Part model, mm, in its own coordinate system. A direction names the side the tool comes from. Give positions to 0.01 mm unless a question says otherwise; leave off trailing zeros. Order: outer loops, then holes, each group sorted by start corner. A loop starts at its lowest first (then second) coordinate and runs counter-clockwise, first axis right, second up. Notation, with made-up numbers: (25, 13.25) - (49, 13.25) arc R16 ccw to (49, 33.25) - close; hole circle Ø11 at (-31, 57.5). An arc over 180 degrees is marked (long way). One line per item, written item: value.
Autodesk Inventor part; units mm, degrees
ref_plane "YZ Plane" through (0, 0, 0) normal (1, 0, 0) x (0, 1, 0)
ref_plane "XZ Plane" through (0, 0, 0) normal (0, 1, 0) x (-1, 0, 0)
ref_plane "XY Plane" through (0, 0, 0) normal (0, 0, 1) x (1, 0, 0)
sketch "Esquisse1" plane through (0, 0, 0) normal (0, 1, 0) x (-1, 0, 0)
  line L0 (35, 35) -> (35, 14)
  line L1 (35, 14) -> (42, 10)
  line L2 (42, 10) -> (42, 0)
  line L3 (35, 35) -> (0, 0)
  line L4 (42, 0) -> (0, 0) construction
  line L5 (35, -35) -> (35, -14)
  line L6 (35, -14) -> (42, -10)
  line L7 (42, -10) -> (42, 0)
  line L8 (35, -35) -> (0, 0)
  line L9 (38.5, -12) -> (38.5, 12) construction
  circle A0 centre (38.5, 0) radius 2.15
  circle A1 centre (38.5, 6) radius 2.15
  circle A2 centre (38.5, -6) radius 2.15
  dimension "d0" = 90
  dimension "d1" = 70
  dimension "d4" = 6
  dimension "d11" = 6
  dimension "d16" = 4.3
  dimension "d17" = 20
  dimension "d18" = 4
  dimension "d19" = 7
extrude "Extrusion1" add sketch "Esquisse1" along normal blind 3
pattern_circular "Réseau circulaire1" count 4 over 360 about axis through (0, 0, 0) along (0, 1, 0) of "Extrusion1"
ref_plane "Plan de construction2" through (0, 0, -14) normal (1, 0, 0) x (0, 0, -1)
ref_plane "Plan de construction3" through (-14, 0, 0) normal (0, 0, -1) x (-1, 0, 0)
chamfer "Chanfrein1" distance 10 angle 45 4 edges at (-35, 1.5, -35) (-35, 1.5, 35) (35, 1.5, -35) (35, 1.5, 35)
sketch "Esquisse3" plane through (0, 0, 0) normal (0, -1, 0) x (1, 0, 0)
  circle A0 centre (0, 38.5) radius 2.15 construction
  circle A1 centre (6, 38.5) radius 2.15 construction
  circle A2 centre (-6, 38.5) radius 2.15 construction
  circle A3 centre (38.5, 6) radius 2.15 construction
  circle A4 centre (38.5, -6) radius 2.15 construction
  circle A5 centre (38.5, 0) radius 2.15 construction
  circle A6 centre (6, -38.5) radius 2.15 construction
  circle A7 centre (-6, -38.5) radius 2.15 construction
  circle A8 centre (0, -38.5) radius 2.15 construction
  circle A9 centre (-38.5, -6) radius 2.15 construction
  circle A10 centre (-38.5, 6) radius 2.15 construction
  circle A11 centre (-38.5, 0) radius 2.15 construction
  line L0 (-35, 25) -> (-35, 14) construction
  line L1 (-35, 14) -> (-42, 10) construction
  line L2 (-42, 10) -> (-42, -10) construction
  line L3 (-42, -10) -> (-35, -14) construction
  line L4 (-35, -14) -> (-35, -25) construction
  line L5 (-25, -35) -> (-14, -35) construction
  line L6 (-14, -35) -> (-10, -42) construction
  line L7 (-10, -42) -> (10, -42) construction
  line L8 (10, -42) -> (14, -35) construction
  line L9 (14, -35) -> (25, -35) construction
  line L10 (35, -25) -> (35, -14) construction
  line L11 (35, -14) -> (42, -10) construction
  line L12 (42, -10) -> (42, 10) construction
  line L13 (42, 10) -> (35, 14) construction
  line L14 (35, 14) -> (35, 25) construction
  line L15 (25, 35) -> (14, 35) construction
  line L16 (14, 35) -> (10, 42) construction
  line L17 (10, 42) -> (-10, 42) construction
  line L18 (-10, 42) -> (-14, 35) construction
  line L19 (-14, 35) -> (-25, 35) construction
  line L20 (-51.72, -12.8291) -> (-12.8291, -51.72)
  line L21 (-12.8291, -51.72) -> (-10, -42)
  line L22 (-42, -10) -> (-51.72, -12.8291)
  line L23 (-35, -14) -> (-42, -10)
  line L24 (-42, -10) -> (-35, -14)
  line L25 (-10, -42) -> (-14, -35)
  line L26 (-14, -35) -> (-10, -42)
  line L27 (25, 35) -> (35, 25)
  line L28 (-35, 25) -> (-25, 35)
  line L29 (-25, -35) -> (-35, -25)
  line L30 (35, -25) -> (25, -35)
  line L31 (-14, -35) -> (-35, -14)
  point P0 (0, 0)
  dimension "d32" = 135
  dimension "d33" = 55
extrude "Extrusion3" add sketch "Esquisse3" against normal blind 3
sketch "Esquisse4" plane through (-51.72, 0, -12.8291) normal (-0.7071068, 0, -0.7071068) x (-0.7071068, 0, 0.7071068)
  line L0 (0, 0) -> (-55, 0) construction
  line L1 (0, 0) -> (0, 3) construction
  line L2 (-55, 3) -> (0, 3) construction
  line L3 (-55, 0) -> (-55, 3) construction
  line L4 (0, 0) -> (-55, 0)
  line L5 (-55, 0) -> (-55, 24)
  line L6 (-55, 24) -> (0, 24)
  line L7 (0, 24) -> (0, 0)
  point P0 (-27.5, 0)
  dimension "d36" = 24
extrude "Extrusion4" add sketch "Esquisse4" along normal blind 3
sketch "Esquisse5" plane through (-53.8413, 0, -14.9504) normal (-0.7071068, 0, -0.7071068) x (-0.7071068, 0, 0.7071068)
  line L0 (-55, 0) -> (0, 0) construction
  line L1 (0, 0) -> (0, 24) construction
  line L2 (0, 24) -> (-55, 24) construction
  line L3 (-55, 24) -> (-55, 0) construction
  line L4 (0, 0) -> (0, 24) construction
  line L5 (0, 9.2801) -> (-55, 9.2801) construction
  circle A0 centre (-15.1412, 9.2801) radius 7.3571
  line L6 (-27.5, 0) -> (-27.5, 24) construction
  circle A1 centre (-39.8588, 9.2801) radius 7.3571
extrude "Extrusion5" cut sketch "Esquisse5" against normal blind 1
pattern_circular "Réseau circulaire2" count 4 over 360 about axis through (0, 0, 0) along (0, -1, 0) of "Extrusion3", "Extrusion4"
fillet "Congé1" radius 3 2 edges at (-34.3959, 0, 34.3959) (34.3959, 0, -34.3959)
sketch "Esquisse6" plane through (0, 0, 0) normal (0, -1, 0) x (1, 0, 0)
  line L0 (51.72, -12.8291) -> (12.8291, -51.72) construction
  line L1 (51.72, -12.8291) -> (42, -10) construction
  line L2 (42, -10) -> (42, 10) construction
  line L3 (42, 10) -> (51.72, 12.8291) construction
  line L4 (51.72, 12.8291) -> (53.8413, 14.9504) construction
  line L5 (14.9504, 53.8413) -> (53.8413, 14.9504) construction
  line L6 (12.8291, 51.72) -> (14.9504, 53.8413) construction
  line L7 (12.8291, 51.72) -> (10, 42) construction
  line L8 (10, 42) -> (-10, 42) construction
  line L9 (-10, 42) -> (-12.8291, 51.72) construction
  line L10 (-51.72, 12.8291) -> (-12.8291, 51.72) construction
  line L11 (-51.72, 12.8291) -> (-42, 10) construction
  line L12 (-42, 10) -> (-42, -10) construction
  line L13 (-42, -10) -> (-51.72, -12.8291) construction
  line L14 (-51.72, -12.8291) -> (-53.8413, -14.9504) construction
  line L15 (-14.9504, -53.8413) -> (-53.8413, -14.9504) construction
  line L16 (-12.8291, -51.72) -> (-14.9504, -53.8413) construction
  line L17 (-12.8291, -51.72) -> (-10, -42) construction
  line L18 (-10, -42) -> (10, -42) construction
  line L19 (10, -42) -> (12.8291, -51.72) construction
  circle A0 centre (0, 38.5) radius 2.15 construction
  circle A1 centre (6, 38.5) radius 2.15 construction
  circle A2 centre (-6, 38.5) radius 2.15 construction
  circle A3 centre (38.5, 6) radius 2.15 construction
  circle A4 centre (38.5, -6) radius 2.15 construction
  circle A5 centre (38.5, 0) radius 2.15 construction
  circle A6 centre (6, -38.5) radius 2.15 construction
  circle A7 centre (-6, -38.5) radius 2.15 construction
  circle A8 centre (0, -38.5) radius 2.15 construction
  circle A9 centre (-38.5, -6) radius 2.15 construction
  circle A10 centre (-38.5, 6) radius 2.15 construction
  circle A11 centre (-38.5, 0) radius 2.15 construction
  line L20 (14.9504, -53.8413) -> (53.8413, -14.9504) construction
  line L21 (22.0215, -46.7702) -> (-16.8694, -7.8793)
  line L22 (-16.8694, -7.8793) -> (7.8793, 16.8694)
  line L23 (7.8793, 16.8694) -> (46.7702, -22.0215)
  line L24 (46.7702, -22.0215) -> (22.0215, -46.7702)
  line L25 (-16.8694, -7.8793) -> (-13.3339, -11.4149) construction
  line L26 (-13.3339, -11.4149) -> (11.4149, 13.3339) construction
  line L27 (11.4149, 13.3339) -> (7.8793, 16.8694) construction
  line L28 (-4.495, 4.495) -> (34.3959, -34.3959) construction
  line L29 (-13.3339, -11.4149) -> (-30.7818, -28.8628) construction
  circle A12 centre (-15.4552, -13.5362) radius 1.7
  circle A13 centre (-18.9907, -17.0717) radius 1.7
  circle A14 centre (13.5362, 15.4552) radius 1.7
  circle A15 centre (17.0717, 18.9907) radius 1.7
  point P0 (0, 0)
  dimension "d48" = 35
  dimension "d49" = 55
  dimension "d54" = 35
  dimension "d69" = 5
  dimension "d70" = 3
  dimension "d71" = 3.4
  dimension "d74" = 5
extrude "Extrusion6" cut sketch "Esquisse6" against normal through all contours L21 L22 L23 L24 keep common part
sketch "Esquisse7" plane through (19.9002, 3, -44.6489) normal (-0.7071068, 0, -0.7071068) x (-0.7071068, 0, 0.7071068)
  circle A0 centre (47, -5.5) radius 3.5
  line L0 (47, -3) -> (47, -5.5) construction
  line L1 (0, -3) -> (52, -3) construction
  point P0 (45.6431, -3)
  point P1 (47, -3)
  dimension "d97" = 2.5
  dimension "d98" = 7
extrude "Extrusion7" add sketch "Esquisse7" against normal blind 35
sketch "Esquisse8" plane through (19.9002, 3, -44.6489) normal (-0.7071068, 0, -0.7071068) x (-0.7071068, 0, 0.7071068)
  arc A0 (43.5, -3) -> (50.5, -3) centre (47, -3) ccw
  line L0 (49.4495, -3) -> (52, -3)
  line L1 (52, -3) -> (52, 0)
  line L2 (52, 0) -> (0, 0)
  line L3 (0, 0) -> (0, 21)
  line L4 (0, 21) -> (-3, 21)
  line L5 (-3, 21) -> (-3, 0)
  arc A1 (-3, 0) -> (0, -3) centre (0, 0) ccw
  line L6 (0, -3) -> (44.5505, -3)
  arc A2 (44.5505, -3) -> (49.4495, -3) centre (47, -5.5) ccw
  arc A3 (44.5505, -3) -> (49.4495, -3) centre (47, -5.5) ccw
  circle A4 centre (47, -5.5) radius 2.3
  point P0 (45.6431, -3)
  dimension "d99" = 4.6
extrude "Extrusion8" cut sketch "Esquisse8" against normal through all contours A4 A0 | A0 A4
sketch "Esquisse11" plane through (19.9002, 3, -44.6489) normal (-0.7071068, 0, -0.7071068) x (-0.7071068, 0, 0.7071068)
  line L0 (49.4495, -3) -> (52, -3)
  line L1 (52, -3) -> (52, 0)
  line L2 (52, 0) -> (0, 0)
  line L3 (0, 0) -> (0, 21)
  line L4 (0, 21) -> (-3, 21)
  line L5 (-3, 21) -> (-3, 0)
  arc A0 (-3, 0) -> (0, -3) centre (0, 0) ccw
  line L6 (0, -3) -> (44.5505, -3)
  arc A1 (44.5505, -3) -> (49.4495, -3) centre (47, -5.5) ccw
  line L7 (49.4495, -3) -> (49, 0) construction
  line L8 (52, 0) -> (0, 0)
  line L9 (49, 0) -> (42, 0) construction
  spline S0 degree 2 poles (49.4495, -3) (49, 0) (42, 0) knots 1 1 1 2 2 2
  point P0 (45.6431, -3)
  dimension "d100" = 3
  dimension "d101" = 10
extrude "Extrusion9" cut sketch "Esquisse11" against normal through all contours A1 L6 A0 L5 L4 L3 L2 S0 keep common part
fillet "Congé4" radius 4 1 edges at (-2.6915, 0, 2.6915)
sketch "Esquisse12" plane through (0, 0, 0) normal (0, -1, 0) x (1, 0, 0)
  line L0 (19.9002, -44.6489) -> (-11.6018, -13.1469)
  line L1 (44.6489, -19.9002) -> (19.9002, -44.6489)
  line L2 (13.1469, 11.6018) -> (44.6489, -19.9002)
  line L3 (22.0215, -46.7702) -> (46.7702, -22.0215) construction
  line L4 (34.3959, -34.3959) -> (-3.4344, 3.4344) construction
  line L5 (-15.8087, -8.94) -> (8.94, 15.8087) construction
  line L6 (-15.8087, -8.94) -> (8.94, 15.8087)
  line L7 (-15.3138, -8.445) -> (22.5165, -46.2752)
  line L8 (8.445, 15.3138) -> (46.2752, -22.5165)
  line L9 (22.5165, -46.2752) -> (22.0215, -46.7702)
  line L10 (22.0215, -46.7702) -> (-15.8087, -8.94)
  line L11 (-15.8087, -8.94) -> (-15.3138, -8.445)
  line L12 (46.2752, -22.5165) -> (46.7702, -22.0215)
  line L13 (46.7702, -22.0215) -> (8.94, 15.8087)
  line L14 (8.94, 15.8087) -> (8.445, 15.3138)
  line L15 (13.1469, 11.6018) -> (-11.6018, -13.1469)
  point P0 (-9.0912, -12.122)
  dimension "d91" = 0.7
extrude "Extrusion10" cut sketch "Esquisse12" along normal through all both and the other way through all contours L0 L15 L7 L1 | L1 L7 L9 L10 | L10 L6 L7 L15 | L8 L15 L2 L1 | L1 L13 L12 L8 | L8 L6 L13 L15
properties part number "clapet"
1) Cut at B-B, the plane y = 19. Give the cut face in (x, z), then the cut area to 3 significant figures.
Outcome:
outline: (20.4, -44.15) - (22.52, -46.28) - (46.28, -22.52) - (44.15, -20.4) - close
area: 101 mm^2
2) Which spindle directions (+Z, -Z, +X, -X, +Y, -Y) get a long thin tool onto all of the face, cutting with end or side? Do faces 5 (the flat face through (6.315, 2.403, -30.074)), 6 (the flat face through (32.44, 13.65, -32.11)). Say none if no direction does.
Outcome:
face 5: -Z, -X, +Y, -Y
face 6: +Z, -X, +Y
3) Cut at C-C, the plane x = 19. Give the cut face in (y, z).
Outcome:
outline: (0, -42.76) - (3, -42.76) - (3, 4.76) - (0, 4.76) - close
4) Cut at A-A, the plane y = -1.5. Give the cut face in (x, z).
Outcome:
outline: (-15.21, -8.55) - (-14.3, -9.46) - (9.46, 14.3) - (8.55, 15.21) - close; (-11.37, -12.38) - (-10.47, -13.29) - (13.29, 10.47) - (12.38, 11.37) - close
5) Mould opens along Z. For faces 1 (the cylindrical face through (-2.628, -3.381, 2.295)), 2 (the flat face through (34.56, 13.65, -34.23)), 3 (the flat face through (18, 3, -23)), 4 (the flat face through (30.074, 2.403, -6.315)) say: released by +Z, released by -Z, zero draft, split by the parting line, or undercut.
Outcome:
face 1: undercut
face 2: released by -Z
face 3: zero draft
face 4: released by +Z
6) Pin check, flat tips, straight feed: pin 1 (1.5 mm diameter, centred on x = -4, y = -0.5, fed in from -Z); pin 2 (6 mm diameter, centred on y = 16.5, z = -29, fed in from -X); pin 3 (1.5 mm diameter, centred on y = -0.5, z = 1.5, fed in from +X). Stop position of each tip, or through.
Outcome:
pin 1: stops at z = -20.32
pin 2: stops at x = 32.55
pin 3: stops at x = 22.82
7) Drill centre lines: line 1 along Y through (x, z) = (11.5, -2); line 2 along X through (y, z) = (-1.5, -5); line 3 along Y through (x, z) = (11, 10). Where is each one in solid material? Low to high. Write a range as from..to.
Outcome:
line 1: y = 0..3
line 2: x = -11.66..-9.85, -3.99..-2.18
line 3: y = -5.33..-3.51, -1.49..2.83
